Verification items for the finished model (mm, model axes). A direction names the side the tool comes from. Round coordinates to 2 decimals unless told otherwise and drop trailing zeros. Loops run counter-clockwise (first coordinate to the right, second up) from the corner with the lowest first, then second, coordinate; pieces in that order, holes last. Notation, with made-up numbers: M -3.5,-31.75 L 3.5,-31.75 A12 ccw 3.5,-24.75 Z; hole C -21,33.25 d5. An arc over 180 degrees is marked long. One line per item, written item: value.
from build123d import *

# Parameters (mm, degrees)
F1_DEPTH = 20
F2_R     = 12
F3_DEPTH = 16.5
F5_DEPTH = 3.5


with BuildPart() as f1:
    # F0 (on Front) → F1 (new body)
    with BuildSketch(Plane.XZ):
        Polygon((0, 20), (0, 0), (20, 0), (40, 0), (40, 3.5), (20, 3.5), (20, 20), align=None)
    extrude(amount=F1_DEPTH)

    # F2 (on face) → F3 (cut, through all)
    with BuildSketch(Plane.XY.offset(20)):
        with Locations((10, -10)):
            Circle(F2_R)
    extrude(amount=-F3_DEPTH, mode=Mode.SUBTRACT)

    # F4 (on face) → F5 (cut, through all)
    with BuildSketch(Plane.XY.offset(3.5)):
        with BuildLine():
            Line((30, -12.75), (35, -12.75))
            ThreePointArc((35, -12.75), (37.75, -10), (35, -7.25))
            Line((35, -7.25), (30, -7.25))
            Line((30, -7.25), (25, -7.25))
            ThreePointArc((25, -7.25), (22.25, -10), (25, -12.75))
            Line((25, -12.75), (30, -12.75))
        make_face()
    extrude(amount=-F5_DEPTH, mode=Mode.SUBTRACT)


solid = f1.part
(1) Depth check by flat-ended pin: pin 1 Ø1 at (x, y) = (21, -11.5) entering from +Z; pin 2 Ø4 at (x, y) = (35, -5.5) entering from -Z; pin 3 Ø2.5 at (y, z) = (-19, 10) entering from +X. Enter the tip coordinate at first touch or a pass-through.
Completed:
pin 1: stops at z = 3.5
pin 2: stops at z = 0
pin 3: stops at x = 20
(2) Mould release check, pull along X, two halves, no side actions. Record for faces 1 (the face through (20, -2, 12)), 2 (the face through (30, -12.75, 2)), 3 (the face through (1, -19, 20)), 4 (the face through (0, -8, 3)): +X half, -X half, draft (parallel to the pull), parting line (faces both ways), or undercut.
Completed:
face 1: +X half
face 2: undercut
face 3: draft
face 4: -X half
(3) Sectioned sample at B-B on z = 11.5. Enter the section's corners in (x, y).
Completed:
outline: M 0,-20 L 3.37,-20 A12 cw 0,-16.63 Z; M 0,-3.37 A12 cw 3.37,0 L 0,0 Z; M 16.63,-20 L 20,-20 L 20,-16.63 A12 cw Z; M 16.63,0 A12 cw 20,-3.37 L 20,0 Z
(4) Sectioned sample at D-D on x = 6. Enter the section's corners in (y, z), and give its area (3 significant figures).
Completed:
outline: M -20,0 L 0,0 L 0,3.5 L -20,3.5 Z
area: 70.0 mm^2
(5) Thickness scan on L1, parallel to Y at x = 28, z = 3.25; L2, parallel to Z at x = 10, y = -2.5; L3, parallel to Y at x = 24, z = 1. Record the ranges inside material, lowest first. Write a range as from..to.
Completed:
L1: y = -20..-12.75, -7.25..0
L2: z = 0..3.5
L3: y = -20..-12.56, -7.44..0
(6) Sectioned sample at A-A on y = -10. Enter the section's corners in (x, z).
Completed:
outline: M 0,0 L 22.25,0 L 22.25,3.5 L 0,3.5 Z; M 37.75,0 L 40,0 L 40,3.5 L 37.75,3.5 Z
(7) Tool access check on faces 5 (the face through (15, -20, 3)), 6 (the face through (18.46, -18.51, 11.87)), 7 (the face through (30, -7.25, 2)). Record the directions out of +Z, -Z, +X, -X, +Y, -Y that give a thin tool (end or side, any length) a straight path to the whole face; none if there is none.
Completed:
face 5: +Z, -Z, +X, -X, -Y
face 6: +Z
face 7: +Z, -Z
(8) Sectioned sample at C-C on x = 24. Enter the section's corners in (y, z), and give its area (3 significant figures).
Completed:
outline: M -20,0 L -12.56,0 L -12.56,3.5 L -20,3.5 Z; M -7.44,0 L 0,0 L 0,3.5 L -7.44,3.5 Z
area: 52.1 mm^2
